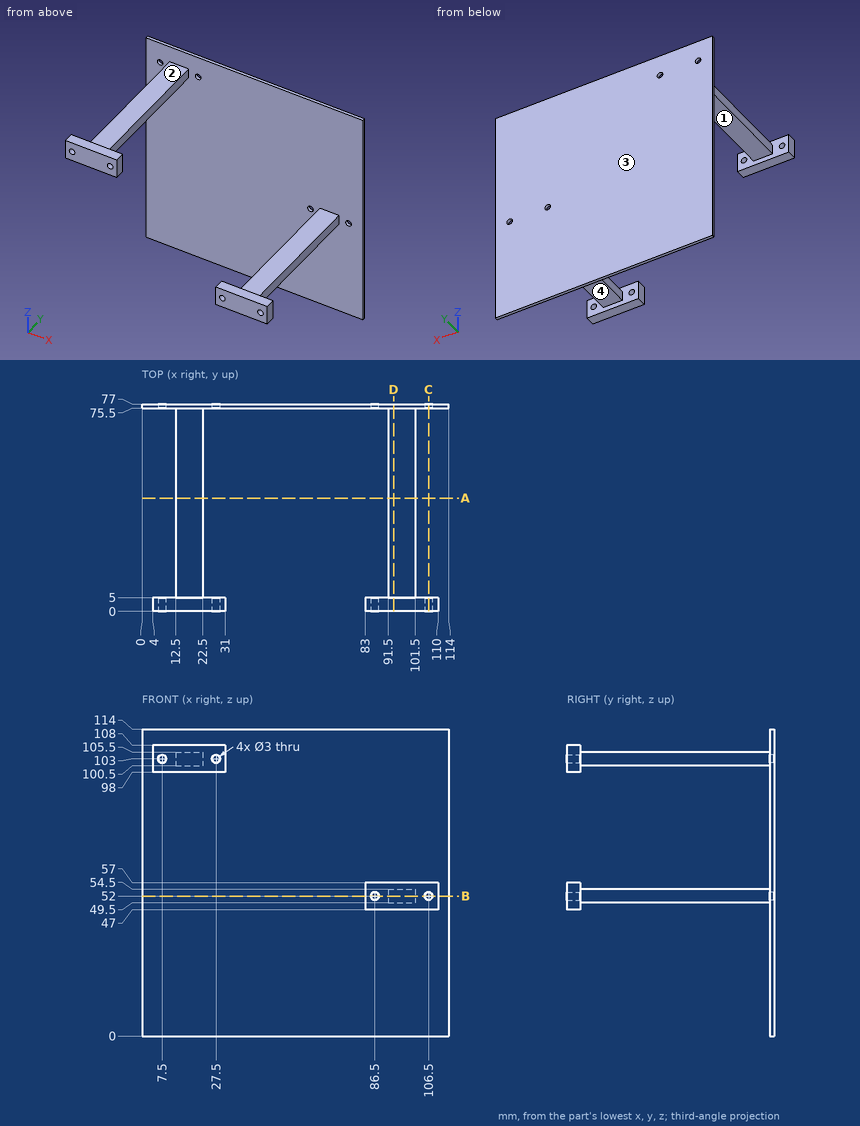
Design review of the part shown in the three views and the two pictorial views. Dimensions are in mm from the part's minimum x, y and z. A direction names the side the tool comes from. Give positions to 0.01 mm unless a question says otherwise; leave off trailing zeros. Loops run counter-clockwise (first coordinate to the right, second up) from the corner with the lowest first, then second, coordinate; pieces in that order, holes last. Notation, with made-up numbers: M -8.5,-39 L 32.5,-39 A24 ccw 32.5,-29 Z; hole C -31,-38.75 d4. An arc over 180 degrees is marked long. Write item = value, one per line.
Q1. To check wall thickness, follow line 1 (X direction, y = 76.65, z = 103); line 2 (X direction, y = 2.15, z = 103); line 3 (Z direction, x = 86.5, y = 3.5). State the ranges of each line that lie inside material, in increasing order. Write a range as [from, to].
Output values:
line_1 = [0, 6], [9, 26], [29, 114]
line_2 = [4, 6], [9, 26], [29, 31]
line_3 = [47, 50.5], [53.5, 57]
Q2. We need section B-B (z = 52). Give the boundary of the cut face in (x, y), plus the area to 3 significant figures.
Output values:
outline = M 0,75.5 L 85,75.5 L 85,77 L 0,77 Z; M 83,0 L 85,0 L 85,5 L 83,5 Z; M 88,0 L 105,0 L 105,5 L 101.5,5 L 101.5,75.5 L 105,75.5 L 105,77 L 88,77 L 88,75.5 L 91.5,75.5 L 91.5,5 L 88,5 Z; M 108,0 L 110,0 L 110,5 L 108,5 Z; M 108,75.5 L 114,75.5 L 114,77 L 108,77 Z
area = 972 mm^2
Q3. Insertion check: pin 1 (2.5 mm diameter, centred on x = 7.5, z = 103, fed in from +Y); pin 2 (4 mm diameter, centred on y = 3, z = 105, fed in from -X); pin 3 (3 mm diameter, centred on x = 22.5, z = 35.5, fed in from -Y); pin 4 (5 mm diameter, centred on x = 19.5, y = 57.5, fed in from -Z). Each pin has a flat end and moves straight along its axis. Give the tip position at first contact, or say it passes through.
Output values:
pin_1 = through
pin_2 = 4
pin_3 = 75.5
pin_4 = 100.5
Q4. We need section C-C (x = 106.5). Give the boundary of the cut face in (y, z).
Output values:
outline = M 0,47 L 5,47 L 5,50.5 L 0,50.5 Z; M 0,53.5 L 5,53.5 L 5,57 L 0,57 Z; M 75.5,0 L 77,0 L 77,50.5 L 75.5,50.5 Z; M 75.5,53.5 L 77,53.5 L 77,114 L 75.5,114 Z
Q5. We need section D-D (x = 93.5). Give the boundary of the cut face in (y, z).
Output values:
outline = M 0,47 L 5,47 L 5,49.5 L 75.5,49.5 L 75.5,0 L 77,0 L 77,114 L 75.5,114 L 75.5,54.5 L 5,54.5 L 5,57 L 0,57 Z
Q6. We need section A-A (y = 42). Give the boundary of the cut face in (x, z).
Output values:
outline = M 12.5,100.5 L 22.5,100.5 L 22.5,105.5 L 12.5,105.5 Z; M 91.5,49.5 L 101.5,49.5 L 101.5,54.5 L 91.5,54.5 Z
Q7. Draft analysis for pull direction Y (two halves, no side actions). For the marked faces 3 and 4, state which applies: +Y half, -Y half, draft (parallel to the pull), parting line (faces both ways), or undercut.
Output values:
face_3 = +Y half
face_4 = undercut
Q8. For the marked faces 1 and 2, list the 3-axis set-ups (+Z, -Z, +X, -X, +Y, -Y) from which the entire face can be reached by the end or side of a thin tool; tool diameter is ignored.
Output values:
face_1 = -Z, +X, -X
face_2 = +Z, +X, -X
